Check sheet for the modelled part. Datum: model origin and axes. Units: mm. Coordinates: 2 decimals unless noted, no trailing zeros.
Autodesk Fusion 360 part; units mm, degrees
sketch "Sketch1" plane through (0, 0, 0) normal (0, 1, 0) x (1, 0, 0)
  circle A0 centre (0, 0) radius 2.1
  line L0 (-6.56, 5.4993) -> (-8.2, 5.4993)
  line L1 (-8.2, 5.4993) -> (-8.2, 3.1)
  line L2 (-8.2, 3.1) -> (-10, 4.9)
  line L3 (-10, 4.9) -> (-10, 10)
  line L4 (-10, 10) -> (-4.9, 10)
  line L5 (-4.9, 10) -> (-3.1, 8.2)
  line L6 (-3.1, 8.2) -> (-5.4993, 8.2)
  line L7 (-5.4993, 8.2) -> (-5.4993, 6.56)
  line L8 (-5.4993, 6.56) -> (-1.7793, 2.84)
  line L9 (-6.56, 5.4993) -> (-2.84, 1.7793)
  line L10 (0, 0) -> (-10, 10) construction
  line L11 (0, 0) -> (0, 5) construction
  line L12 (0, 0) -> (-5, 0) construction
  line L13 (-2.84, 1.7793) -> (-2.84, 0)
  line L14 (-1.7793, 2.84) -> (0, 2.84)
  line L15 (-8.2, -3.1) -> (-10, -4.9)
  line L16 (-6.56, -5.4993) -> (-8.2, -5.4993)
  line L17 (-10, -4.9) -> (-10, -10)
  line L18 (-4.9, -10) -> (-3.1, -8.2)
  line L19 (-5.4993, -6.56) -> (-1.7793, -2.84)
  line L20 (-6.56, -5.4993) -> (-2.84, -1.7793)
  line L21 (-1.7793, -2.84) -> (0, -2.84)
  line L22 (-3.1, -8.2) -> (-5.4993, -8.2)
  line L23 (-8.2, -5.4993) -> (-8.2, -3.1)
  line L24 (-10, -10) -> (-4.9, -10)
  line L25 (-5.4993, -8.2) -> (-5.4993, -6.56)
  line L26 (-2.84, -1.7793) -> (-2.84, 0)
  line L27 (4.9, 10) -> (3.1, 8.2)
  line L28 (2.84, -1.7793) -> (2.84, 0)
  line L29 (6.56, -5.4993) -> (2.84, -1.7793)
  line L30 (1.7793, 2.84) -> (0, 2.84)
  line L31 (5.4993, -8.2) -> (5.4993, -6.56)
  line L32 (5.4993, -6.56) -> (1.7793, -2.84)
  line L33 (10, 10) -> (4.9, 10)
  line L34 (2.84, 1.7793) -> (2.84, 0)
  line L35 (3.1, 8.2) -> (5.4993, 8.2)
  line L36 (10, -10) -> (4.9, -10)
  line L37 (1.7793, -2.84) -> (0, -2.84)
  line L38 (5.4993, 6.56) -> (1.7793, 2.84)
  line L39 (4.9, -10) -> (3.1, -8.2)
  line L40 (6.56, 5.4993) -> (2.84, 1.7793)
  line L41 (5.4993, 8.2) -> (5.4993, 6.56)
  line L42 (3.1, -8.2) -> (5.4993, -8.2)
  line L43 (10, -4.9) -> (10, 4.9) construction
  line L44 (20, 0) -> (30, 10) construction
  line L45 (26.56, -5.4993) -> (28.2, -5.4993)
  line L46 (23.1, 8.2) -> (25.4993, 8.2)
  line L47 (30, 4.9) -> (30, 10)
  line L48 (26.56, 5.4993) -> (22.84, 1.7793)
  line L49 (22.84, -1.7793) -> (22.84, 0)
  line L50 (30, -4.9) -> (30, -10)
  line L51 (25.4993, -8.2) -> (25.4993, -6.56)
  line L52 (23.1, -8.2) -> (25.4993, -8.2)
  line L53 (28.2, 5.4993) -> (28.2, 3.1)
  line L54 (28.2, 3.1) -> (30, 4.9)
  line L55 (20, 0) -> (20, 5) construction
  line L56 (20, 0) -> (25, 0) construction
  line L57 (30, -10) -> (24.9, -10)
  line L58 (26.56, -5.4993) -> (22.84, -1.7793)
  line L59 (24.9, -10) -> (23.1, -8.2)
  line L60 (25.4993, 8.2) -> (25.4993, 6.56)
  line L61 (28.2, -3.1) -> (30, -4.9)
  line L62 (22.84, 1.7793) -> (22.84, 0)
  line L63 (28.2, -5.4993) -> (28.2, -3.1)
  line L64 (10, -10) -> (15.1, -10)
  line L65 (16.9, 8.2) -> (14.5007, 8.2)
  line L66 (18.2207, 2.84) -> (20, 2.84)
  line L67 (14.5007, -6.56) -> (18.2207, -2.84)
  line L68 (15.1, 10) -> (16.9, 8.2)
  line L69 (13.44, 5.4993) -> (17.16, 1.7793)
  line L70 (18.2207, -2.84) -> (20, -2.84)
  line L71 (17.16, 1.7793) -> (17.16, 0)
  line L72 (15.1, -10) -> (16.9, -8.2)
  line L73 (14.5007, 6.56) -> (18.2207, 2.84)
  line L74 (17.16, -1.7793) -> (17.16, 0)
  line L75 (21.7793, 2.84) -> (20, 2.84)
  line L76 (30, 10) -> (24.9, 10)
  line L77 (26.56, 5.4993) -> (28.2, 5.4993)
  line L78 (24.9, 10) -> (23.1, 8.2)
  line L79 (25.4993, -6.56) -> (21.7793, -2.84)
  line L80 (14.5007, 8.2) -> (14.5007, 6.56)
  line L81 (10, 10) -> (15.1, 10)
  circle A1 centre (20, 0) radius 2.1
  line L82 (14.5007, -8.2) -> (14.5007, -6.56)
  line L83 (21.7793, -2.84) -> (20, -2.84)
  line L84 (16.9, -8.2) -> (14.5007, -8.2)
  line L85 (25.4993, 6.56) -> (21.7793, 2.84)
  line L86 (13.44, -5.4993) -> (17.16, -1.7793)
  line L87 (6.56, 5.4993) -> (7.2993, 6.2387)
  line L88 (7.2993, 6.2387) -> (7.2993, 8.2)
  line L89 (7.2993, 8.2) -> (12.7007, 8.2)
  line L90 (12.7007, 8.2) -> (12.7007, 6.2387)
  line L91 (12.7007, 6.2387) -> (13.44, 5.4993)
  line L92 (6.56, -5.4993) -> (7.2993, -6.2387)
  line L93 (7.2993, -6.2387) -> (7.2993, -8.2)
  line L94 (7.2993, -8.2) -> (12.7007, -8.2)
  line L95 (12.7007, -8.2) -> (12.7007, -6.2387)
  line L96 (12.7007, -6.2387) -> (13.44, -5.4993)
  point P0 (5, 0)
  point P1 (15, 0)
  point P2 (20, 0)
  point P3 (20, 0)
  dimension "d1" = 4.2
  dimension "d2" = 10
  dimension "d3" = 10
  dimension "d4" = 3.1
  dimension "d5" = 1.8
  dimension "d6" = 0
  dimension "d7" = 1.5
  dimension "d8" = 1.64
  dimension "d9" = 135
  dimension "d10" = 0
  dimension "d11" = 2.84
  dimension "d12" = 0
  dimension "d13" = 0
  dimension "d14" = 20
  dimension "d15" = 0
  dimension "d16" = 0
extrude "Extrude1" add sketch "Sketch1" along normal mid plane 520
equation "d4 = ( 6.2 / 2 ) * 1 mm"
equation "d6 = d10"
equation "d10 = d9"
equation "d11 = ( 5.68 / 2 ) * 1 mm"
equation "d12 = d19"
equation "d13 = d13"
equation "d15 = d10"
equation "d16 = d29"
1) Scan lines: line 1 (X direction, y = 98.5, z = 0); line 2 (X direction, y = -237, z = -6.5); line 3 (Z direction, x = 25, y = -62). Record each from-to range of solid material in increasing order.
Answer sheet:
line 1: x = -2.84 to -2.1, 2.1 to 2.84, 17.16 to 17.9, 22.1 to 22.84
line 2: x = -10 to -5.44, 5.44 to 7.3, 12.7 to 14.56, 25.44 to 30
line 3: z = -10 to -8.2, -6.06 to -3.94, 3.94 to 6.06, 8.2 to 10
2) Depth check by flat-ended pin: pin 1 (3 mm diameter, centred on x = 0, y = 113.5, fed in from -Z); pin 2 (1.2 mm diameter, centred on x = 4, y = 37.5, fed in from -Z); pin 3 (4 mm diameter, centred on x = -0.5, y = 25.5, fed in from +Z). Enter the tip coordinate at first touch or a pass-through.
Answer sheet:
pin 1: stops at z = -2.84
pin 2: stops at z = -9.7
pin 3: stops at z = 3.56
3) Section check A-A on y = -9. Give the number of separate pieces and of enclosed holes in the cut face, plus the area to 3 significant figures.
Answer sheet:
separate pieces: 1
enclosed holes: 3
area: 255 mm2
